from build123d import *

# Parameters (mm, degrees)
SKETCH_1_W          = 20
SKETCH_1_H          = 20
EXTRUDE_1_DEPTH     = 54
FILLET_1_R          = 1
SKETCH_2_W          = 1
SKETCH_2_H          = 20
CUT_EXTRUDE_1_DEPTH = 1


with BuildPart() as part:
    # 草图1 → 凸台-拉伸1 (new body)
    with BuildSketch(Plane(origin=(0, 0, 0), x_dir=(1, 0, 0), z_dir=(0, 1, 0))):
        with Locations((10, 10)):
            Rectangle(SKETCH_1_W, SKETCH_1_H)
    extrude(amount=EXTRUDE_1_DEPTH)

    # 圆角1
    fillet_1_edges = [part.edges().sort_by_distance(p)[0] for p in [
        (0, 27, -20),
        (20, 27, -20),
        (20, 27, 0),
        (0, 27, 0),
    ]]
    fillet(fillet_1_edges, radius=FILLET_1_R)

    # 草图2 → 切除-拉伸1 (cut)
    with BuildSketch(Plane(origin=(0, 54, 0), x_dir=(1, 0, 0), z_dir=(0, 1, 0))):
        with Locations((10, 10)):
            Rectangle(SKETCH_2_W, SKETCH_2_H)
    extrude(amount=-CUT_EXTRUDE_1_DEPTH, mode=Mode.SUBTRACT)


solid = part.part
Here's how the part is built. I have some questions about the finished solid (model axes, mm). A direction names the side the tool comes from. Give positions to 0.01 mm unless a question says otherwise; leave off trailing zeros. One line per item, written item: value. Start each with the question number.
1. For faces 4 (the face through (19.715, 27.378, -19.699)), 5 (the face through (10.5, 53.5, -9.9)), which set-ups out of +Z, -Z, +X, -X, +Y, -Y let a thin tool reach every point of the face, with its end or its side?
2. Will this pin go through, and if not, where does the flat tip stop? pin 1 Ø0.5 at (x, z) = (10, -9.5) entering from +Y.
3. We'd pull the mould along X, two halves only. Please class faces 1 (the face through (10, 53, -10)), 2 (the face through (20, 27, -10)), 3 (the face through (10, 27, -20)): released by +X, released by -X, zero draft, split by the parting line, or undercut.
Values follow:
1. face 4: -Z, +X, +Y, -Y
1. face 5: +Z, -Z, +Y
2. pin 1: stops at y = 53
3. face 1: undercut
3. face 2: released by +X
3. face 3: zero draft
